Read the model definition and answer for the solid it produces. Units are mm, in the model's axes. Face numbers are marked on the shaded views. A direction names the side the tool comes from. Round coordinates to 2 decimals unless told otherwise and drop trailing zeros. Order: outer loops, then holes, each group sorted by start corner. A loop starts at its lowest first (then second) coordinate and runs counter-clockwise, first axis right, second up. Notation, with made-up numbers: (22, 81) -> (54, 81) arc R30 cw to (54, 115) -> close; hole circle Ø11 at (46.5, -23). An arc over 180 degrees is marked (long way). Use a Markdown table: item, result. Add a question column.
1. Section B-B, the plane z = -8.75 is taken. Give the vertices of the cut face in (x, y), then the cut area to 3 significant figures.
2. Consider L1, parallel to X at y = 10.5, z = -3.5; L2, parallel to Z at x = 5.5, y = 4.25; L3, parallel to Z at x = 12.25, y = 10.25. Determine where each line is inside the solid, lowest interval first. Write a range as [from, to].
3. Given pin 1 (3 mm diameter, centred on x = 7.5, z = -12.5, fed in from +Y), flat-ended and moving along its own axis, determine where the tip first touches the part or whether it passes through.
4. For the marked faces 1 and 2, determine the directions among +Z, -Z, +X, -X, +Y, -Y from which every point of the face is accessible in a straight line to the end or side of a thin tool.
5. The mould has two halves that part along X. Classify the marked faces 3, 4, 5 and 6: +X half, -X half, draft (parallel to the pull), parting line (faces both ways), or undercut.
6. Section D-D, the plane x = 0 is taken. Give the vertices of the cut face in (y, z), then the cut area to 3 significant figures.
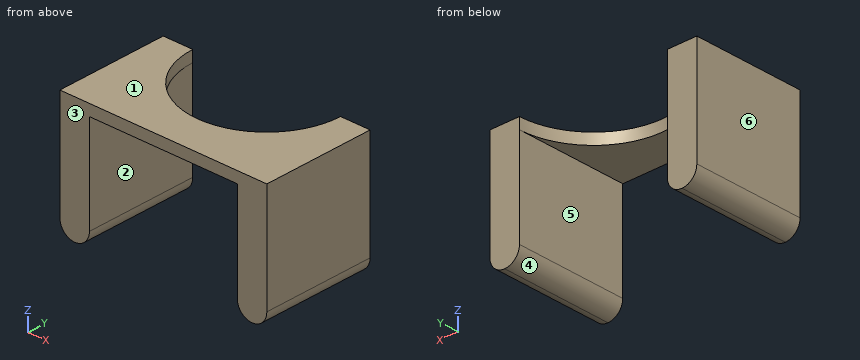
Autodesk Inventor part; units mm, degrees
ref_plane "YZ Plane" through (0, 0, 0) normal (1, 0, 0) x (0, 1, 0)
ref_plane "XZ Plane" through (0, 0, 0) normal (0, 1, 0) x (-1, 0, 0)
ref_plane "XY Plane" through (0, 0, 0) normal (0, 0, 1) x (1, 0, 0)
sketch "Sketch1" plane through (0, 0, 0) normal (0, 1, 0) x (-1, 0, 0)
  line L0 (14, 0) -> (-14, 0)
  line L1 (0, -18.3) -> (0, 4.8)
  line L2 (14, 1.5) -> (-14, 1.5)
  line L3 (-14, 1.5) -> (-14, 0)
  line L4 (-10, 0) -> (10, 0)
  line L5 (14, 0) -> (14, 1.5)
  line L6 (10, 0) -> (10, -15)
  line L7 (10, -15) -> (14, -15)
  line L8 (14, -15) -> (14, 0)
  line L9 (-10, 0) -> (-10, -15)
  line L10 (-10, -15) -> (-14, -15)
  line L11 (-14, -15) -> (-14, 0)
  point P0 (0, 0)
  dimension "d0" = 28
  dimension "d1" = 4
  dimension "d2" = 15
  dimension "d3" = 1.5
  dimension "d5" = 4
  dimension "d6" = 15
extrude "Extrusion1" add sketch "Sketch1" along normal blind 15
fillet "Fillet1" radius 2 4 edges at (14, 7.5, -15) (10, 7.5, -15) (-10, 7.5, -15) (-14, 7.5, -15)
sketch "Sketch2" plane through (-14, 0, 1.5) normal (0, 0, 1) x (1, 0, 0)
  line L0 (0, 0) -> (28, 0)
  line L1 (28, 0) -> (28, 15)
  line L2 (0, 15) -> (28, 15)
  line L3 (0, 0) -> (0, 15)
  line L4 (24, 0) -> (24, 15)
  line L5 (4, 0) -> (4, 15)
  circle A0 centre (14, 15) radius 10
  point P0 (14, 0)
extrude "Extrusion2" cut sketch "Sketch2" against normal blind 15 contours A0 L2 | L2 A0
properties part number "encastre pinza pilar central"
Verdict:
| question | item | result |
|---|---|---|
| 1 | outline | (-14, 0) -> (-10, 0) -> (-10, 15) -> (-14, 15) -> close; (10, 0) -> (14, 0) -> (14, 15) -> (10, 15) -> close |
| 1 | area | 120 mm2 |
| 2 | L1 | x = [-14, -10], [10, 14] |
| 2 | L2 | z = [0, 1.5] |
| 2 | L3 | z = [-14.98, 1.5] |
| 3 | pin 1 | passes through |
| 4 | face 1 | +Z, +X, -X, +Y, -Y |
| 4 | face 2 | -Z, +Y, -Y |
| 5 | face 3 | draft |
| 5 | face 4 | undercut |
| 5 | face 5 | undercut |
| 5 | face 6 | -X half |
| 6 | outline | (0, 0) -> (5, 0) -> (5, 1.5) -> (0, 1.5) -> close |
| 6 | area | 7.50 mm2 |
